Autodesk Inventor part; units mm, degrees
ref_plane "YZ Plane" through (0, 0, 0) normal (1, 0, 0) x (0, 1, 0)
ref_plane "XZ Plane" through (0, 0, 0) normal (0, 1, 0) x (-1, 0, 0)
ref_plane "XY Plane" through (0, 0, 0) normal (0, 0, 1) x (1, 0, 0)
sketch "Sketch1" plane through (0, 0, 0) normal (0, 1, 0) x (-1, 0, 0)
  line L0 (0, 0) -> (0, -90)
  line L1 (0, -90) -> (56, -90)
  line L2 (56, -90) -> (56, 0)
  line L3 (56, 0) -> (0, 0)
  dimension "d0" = 90
  dimension "d1" = 56
extrude "Extrusion1" add sketch "Sketch1" along normal blind 4
sketch "Sketch2" plane through (0, 4, 0) normal (0, 1, 0) x (1, 0, 0)
  circle A0 centre (-3, 3) radius 3
  circle A1 centre (-52.9351, 2.9993) radius 3
  circle A2 centre (-53, 87) radius 3
  circle A3 centre (-3, 87) radius 3
  point P0 (0, 0)
  point P1 (-56, 0)
  point P2 (0, 90)
  point P3 (-56, 90)
  dimension "d6" = 6
  dimension "d17" = 6
  dimension "d20" = 6
  dimension "d23" = 6
sketch "Sketch5" plane through (0, 0, -90) normal (0, 0, -1) x (-1, 0, 0)
  line L0 (0, 0) -> (56, 0)
  line L1 (0, 0) -> (56, 0)
  line L2 (56, 0) -> (56, 4)
  line L3 (56, 0) -> (56, 4)
  line L4 (56, 4) -> (0, 4)
  line L5 (0, 0) -> (0, 4)
  line L6 (0, 0) -> (0, 4)
extrude "Extrusion2" add sketch "Sketch5" along normal blind 1
sketch "Sketch7" plane through (-56, 0, 0) normal (0, 0, 1) x (1, 0, 0)
  line L0 (0, 0) -> (0, 4)
  line L1 (0, 4) -> (0, 0)
  line L2 (0, 0) -> (56, 0)
  line L3 (56, 0) -> (56, 4)
  line L4 (56, 4) -> (0, 4)
extrude "Extrusion3" add sketch "Sketch7" along normal blind 1
sketch "Sketch8" plane through (0, 0, -91) normal (1, 0, 0) x (0, 0, -1)
  line L0 (-92, 0) -> (-92, 4)
  line L1 (0, 0) -> (-92, 0)
  line L2 (-92, 4) -> (-92, 0)
  line L3 (-92, 0) -> (0, 0)
  line L4 (0, 4) -> (0, 0)
  line L5 (0, 0) -> (0, 4)
  line L6 (0, 4) -> (-92, 4)
  line L7 (0, 4) -> (-92, 4)
  point P0 (-91, 0)
extrude "Extrusion4" add sketch "Sketch8" along normal blind 1
sketch "Sketch9" plane through (-56, 0, -91) normal (-1, 0, 0) x (0, 0, 1)
  line L0 (92, 0) -> (0, 0)
  line L1 (92, 4) -> (92, 0)
  line L2 (0, 0) -> (92, 0)
  line L3 (92, 0) -> (92, 4)
  line L4 (92, 4) -> (0, 4)
  line L5 (0, 4) -> (0, 0)
  point P0 (91, 0)
extrude "Extrusion5" add sketch "Sketch9" along normal blind 1
sketch "Sketch10" plane through (1, 0, -91) normal (1, 0, 0) x (0, 0, -1)
  point P0 (-91, 0)
extrude "Extrusion6" cut sketch "Sketch2" against normal blind 2
sketch "Sketch11" plane through (-3, 2, -87) normal (0, 1, 0) x (1, 0, 0)
  circle A0 centre (0, -84) radius 3
  circle A1 centre (0, -84) radius 1.6
  circle A2 centre (-49.9351, -84.0007) radius 3
  circle A3 centre (-49.9351, -84.0007) radius 1.6
  circle A4 centre (-50, 0) radius 3
  circle A5 centre (-50, 0) radius 1.6
  circle A6 centre (0, 0) radius 3
  circle A7 centre (0, 0) radius 1.6
  point P0 (3, -87)
  dimension "d26" = 3.2
  dimension "d27" = 3.2
  dimension "d28" = 3.2
  dimension "d29" = 3.2
extrude "Extrusion7" cut sketch "Sketch11" against normal blind 2 contours A1 | A3 | A5 | A7
sketch "Sketch12" plane through (0, 4, 0) normal (0, 1, 0) x (1, 0, 0)
  line L0 (-47, 9) -> (-47, 24)
  line L1 (-47, 24) -> (-32, 24)
  line L2 (-32, 24) -> (-32, 9)
  line L3 (-32, 9) -> (-47, 9)
  line L4 (-47, 30) -> (-32, 30)
  line L5 (-32, 30) -> (-32, 45)
  line L6 (-32, 45) -> (-47, 45)
  line L7 (-47, 45) -> (-47, 30)
  line L8 (-47, 51) -> (-47, 66)
  line L9 (-47, 66) -> (-32, 66)
  line L10 (-32, 66) -> (-32, 51)
  line L11 (-32, 51) -> (-47, 51)
  line L12 (-57, 91) -> (1, 91)
  line L13 (-26, 9) -> (-26, 24)
  line L14 (-26, 24) -> (-11, 24)
  line L15 (-11, 24) -> (-11, 9)
  line L16 (-11, 9) -> (-26, 9)
  circle A0 centre (-18.5, 34) radius 3
  circle A1 centre (-18.5, 54) radius 3
  circle A2 centre (-18.5, 74) radius 3
  line L17 (-18.5, 54) -> (-18.5, 74)
  point P0 (0, 0)
  point P1 (-57, -1)
  dimension "d34" = 15
  dimension "d35" = 15
  dimension "d37" = 15
  dimension "d39" = 15
  dimension "d44" = 15
  dimension "d46" = 6
  dimension "d48" = 6
  dimension "d50" = 6
  dimension "d57" = 20
extrude "Extrusion8" cut sketch "Sketch12" against normal blind 4
sketch "Sketch13" plane through (0, 4, 0) normal (0, 1, 0) x (1, 0, 0)
  circle A0 centre (-18.5, 34) radius 3
  circle A1 centre (-18.5, 34) radius 7.5
  circle A2 centre (-18.5, 54) radius 3
  circle A3 centre (-18.5, 54) radius 7.5
  circle A4 centre (-18.5, 74) radius 3
  circle A5 centre (-18.5, 74) radius 7.5
  point P0 (0, 0)
  dimension "d58" = 15
  dimension "d59" = 15
  dimension "d60" = 15
extrude "Extrusion9" cut sketch "Sketch13" against normal blind 1
properties part number "streamdeck lid"
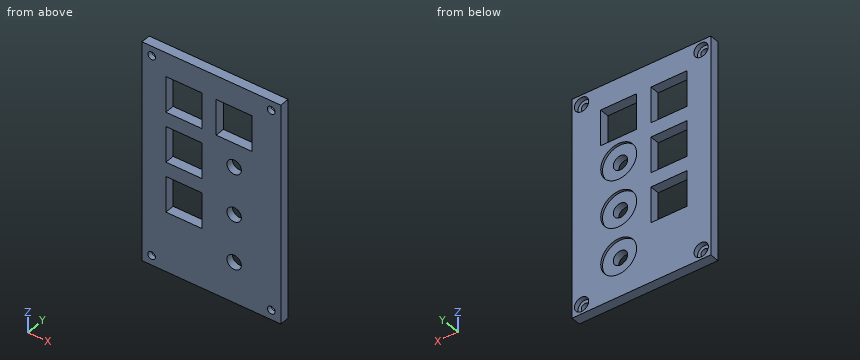
CAD build for the part. Positions are in the model's coordinates, mm. Round coordinates to 2 decimals unless told otherwise and drop trailing zeros. Write each loop counter-clockwise with the first axis right and the second up, starting at its lowest first coordinate (ties: lowest second). Pieces come first, ordered by that corner, then holes. Notation, with made-up numbers: (14, -27) - (24, -27) arc R14 cw to (24, -11) - close; hole circle Ø3 at (19, 61.25). An arc over 180 degrees is marked (long way). Return JSON: item names as keys, results as strings. Group by question number.
Item 1: Band-saw the part on A-A on z = -87. List the corners of the cut face in (x, y), plus the area to 3 significant figures.
Item 2: Probe probe 1 along Z at (x, y) = (-45, 1.85); probe 2 along Z at (x, y) = (-53, 1); probe 3 along Z at (x, y) = (-18.5, 1.1). List the from-to ranges inside material, lowest first.
Item 3: Band-saw the part on C-C on z = -74. List the corners of the cut face in (x, y), plus the area to 3 significant figures.
Item 4: Band-saw the part on D-D on x = -39.5. List the corners of the cut face in (y, z).
Item 5: Flat gauge pin, fed straight in: pin 1 Ø3.5 at (x, z) = (-53, -87) entering from +Y. Where does the tip first touch, or does it go through?
Item 6: Band-saw the part on B-B on x = -18.5. State how many separate pieces and enclosed holes the cut face has, plus the area to 3 significant figures.
Resolved:
{
 "1": {"outline": "(-57, 0) - (-54.6, 0) - (-54.6, 2) - (-56, 2) - (-56, 4) - (-57, 4) - close; (-51.4, 0) - (-4.6, 0) - (-4.6, 2) - (-6, 2) - (-6, 4) - (-50, 4) - (-50, 2) - (-51.4, 2) - close; (-1.4, 0) - (1, 0) - (1, 4) - (0, 4) - (0, 2) - (-1.4, 2) - close", "area": "195 mm²"},
 "2": {"probe 1": "z = -91 to -66, -51 to -45, -30 to -24, -9 to 1", "probe 2": "z = -91 to -88.6, -85.4 to -4.6, -1.4 to 1", "probe 3": "z = -91 to -77, -71 to -57, -51 to -37, -31 to -24, -9 to 1"},
 "3": {"outline": "(-57, 0) - (-21.5, 0) - (-21.5, 3) - (-26, 3) - (-26, 4) - (-57, 4) - close; (-15.5, 0) - (1, 0) - (1, 4) - (-11, 4) - (-11, 3) - (-15.5, 3) - close", "area": "199 mm²"},
 "4": {"outline": "(0, -91) - (4, -91) - (4, -66) - (0, -66) - close; (0, -51) - (4, -51) - (4, -45) - (0, -45) - close; (0, -30) - (4, -30) - (4, -24) - (0, -24) - close; (0, -9) - (4, -9) - (4, 1) - (0, 1) - close"},
 "5": {"pin 1": "stops at y = 2"},
 "6": {"separate pieces": "5", "enclosed holes": "0", "area": "209 mm²"}
}
